Part model, mm, in its own coordinate system. A direction names the side the tool comes from. Coordinates: 2 decimals unless noted, no trailing zeros. Loops run counter-clockwise (first coordinate to the right, second up) from the corner with the lowest first, then second, coordinate; pieces in that order, holes last. Notation, with made-up numbers: (9.5, 2.5) - (54.5, 2.5) arc R20 ccw to (54.5, 27.5) - close; hole circle Ø3 at (34.25, 15.25). An arc over 180 degrees is marked (long way). Use a Markdown table: item, result. Add a question column.
1. Pull direction X, two halves, no side cores. Call faces 1 (the flat face through (64.044, -34.015, -2.576)), 2 (the flat face through (35, -32.512, -32)), 3 (the cylindrical face through (58.546, -34.015, -52.371)): pulls with the +X half, pulls with the -X half, needs draft (parallel to the pull), parting line crosses it, or undercut.
2. Wall check: probe 1 along X at (y, z) = (11.5, -4); probe 2 along Y at (x, z) = (9.5, -21); probe 3 along X at (y, z) = (-32, -7.5). Give the ranges that are in metal, low to high. Write a range as [from, to].
3. Band-saw the part on C-C, the plane y = 0. Give the cut face in (x, z).
4. Band-saw the part on A-A, the plane z = -32.5. Give the cut face in (x, y), plus the area to 3 significant figures.
5. Drop flat-ended pins along their axis: pin 1 (6 mm diameter, centred on y = -20, z = -29.5, fed in from +X); pin 2 (10 mm diameter, centred on x = 43, z = -43.5, fed in from +Y). Give the stop position or say it passes through.
6. 3-axis set-ups, long thin cutter, end or side, ignore diameter. For faces 4 (the flat face through (1.524, -12, -47)), 5 (the cylindrical face through (12.574, -34.015, -12.399)), 6 (the cylindrical face through (0, 25.7, -58.2)): which of +Z, -Z, +X, -X, +Y, -Y reach the whole face in a straight line?
7. Band-saw the part on D-D, the plane y = 17.5. Give the cut face in (x, z), plus the area to 3 significant figures.
8. Band-saw the part on B-B, the plane x = 48.5. Give the cut face in (y, z) (3 decimals), plus the area to 3 significant figures.
from build123d import *

# Parameters (mm, degrees)
BOSS_EXTRUDE1_DEPTH = 65.024
CUT_EXTRUDE1_DEPTH  = 65.024
SKETCH3_R           = 19.05
SKETCH3_R_2         = 2.794
CUT_EXTRUDE2_DEPTH  = 65.024
FILLET1_R           = 2.54
CHAMFER1_SIZE       = 5.08


with BuildPart() as part:
    # Sketch1 → Boss-Extrude1 (new body)
    with BuildSketch(Plane.XY):
        Polygon((-1.524, 32.512), (1.524, 32.512), (1.524, -32.512), (66.548, -32.512), (66.548, -35.56), (-1.524, -35.56), (-1.524, -32.512), align=None)
    extrude(amount=-BOSS_EXTRUDE1_DEPTH)

    # Sketch2 → Cut-Extrude1 (cut)
    with BuildSketch(Plane(origin=(0, -32.512, 0), x_dir=(1, 0, 0), z_dir=(0, 1, 0))):
        with BuildLine():
            Line((14.732, 14.605), (56.388, 14.605))
            ThreePointArc((56.388, 14.605), (58.547, 12.446), (56.388, 10.287))
            Line((56.388, 10.287), (14.732, 10.287))
            ThreePointArc((14.732, 10.287), (12.573, 12.446), (14.732, 14.605))
        make_face()
        with BuildLine():
            Line((14.732, 54.483), (56.388, 54.483))
            ThreePointArc((56.388, 54.483), (58.547, 52.324), (56.388, 50.165))
            Line((56.388, 50.165), (14.732, 50.165))
            ThreePointArc((14.732, 50.165), (12.573, 52.324), (14.732, 54.483))
        make_face()
    extrude(amount=-CUT_EXTRUDE1_DEPTH, mode=Mode.SUBTRACT)

    # Sketch3 → Cut-Extrude2 (cut)
    with BuildSketch(Plane.ZY.offset(1.524)):
        with Locations((-32.512, 3.556)):
            Circle(SKETCH3_R)
        with Locations((-56.007, -18.288)):
            Circle(SKETCH3_R_2)
        with Locations((-9.017, -18.288)):
            Circle(SKETCH3_R_2)
        with Locations((-9.017, 27.432)):
            Circle(SKETCH3_R_2)
        with Locations((-56.007, 27.432)):
            Circle(SKETCH3_R_2)
    extrude(amount=-CUT_EXTRUDE2_DEPTH, mode=Mode.SUBTRACT)

    # Fillet1
    fillet1_edges = [part.edges().sort_by_distance(p)[0] for p in [
        (1.524, -32.512, -32.512),
    ]]
    fillet(fillet1_edges, radius=FILLET1_R)

    # Chamfer1
    chamfer1_edges = [part.edges().sort_by_distance(p)[0] for p in [
        (0, 32.512, -65.024),
        (66.548, -34.036, -65.024),
        (66.548, -34.036, 0),
        (0, 32.512, 0),
    ]]
    chamfer(chamfer1_edges, length=CHAMFER1_SIZE)


solid = part.part
Geometry check:
| question | item | result |
|---|---|---|
| 1 | face 1 | pulls with the +X half |
| 1 | face 2 | needs draft |
| 1 | face 3 | undercut |
| 2 | probe 1 | x = [-1.52, 1.52] |
| 2 | probe 2 | y = [-35.56, -32.51] |
| 2 | probe 3 | x = [-1.52, 2.53] |
| 3 | outline | (-1.52, -65.02) - (1.52, -65.02) - (1.52, -51.23) - (-1.52, -51.23) - close; (-1.52, -13.8) - (1.52, -13.8) - (1.52, 0) - (-1.52, 0) - close |
| 4 | outline | (-1.52, -35.56) - (66.55, -35.56) - (66.55, -32.51) - (4.06, -32.51) arc R2.54 cw to (1.52, -29.97) - (1.52, -15.49) - (-1.52, -15.49) - close; (-1.52, 22.61) - (1.52, 22.61) - (1.52, 32.51) - (-1.52, 32.51) - close |
| 4 | area | 291 mm^2 |
| 5 | pin 1 | stops at x = 1.52 |
| 5 | pin 2 | stops at y = -32.51 |
| 6 | face 4 | +Z, -Z, +X, +Y |
| 6 | face 5 | +Y, -Y |
| 6 | face 6 | +X, -X |
| 7 | outline | (-1.52, -65.02) - (1.52, -65.02) - (1.52, -45.49) - (-1.52, -45.49) - close; (-1.52, -19.53) - (1.52, -19.53) - (1.52, 0) - (-1.52, 0) - close |
| 7 | area | 119 mm^2 |
| 8 | outline | (-35.56, -65.024) - (-32.512, -65.024) - (-32.512, -54.483) - (-35.56, -54.483) - close; (-35.56, -50.165) - (-32.512, -50.165) - (-32.512, -14.605) - (-35.56, -14.605) - close; (-35.56, -10.287) - (-32.512, -10.287) - (-32.512, 0) - (-35.56, 0) - close |
| 8 | area | 172 mm^2 |
